For this review, use the dimensioned drawing (mm, ordinates from the lowest corner) and the shaded views. A direction names the side the tool comes from. Round coordinates to 2 decimals unless told otherwise and drop trailing zeros. Loops run counter-clockwise (first coordinate to the right, second up) from the corner with the lowest first, then second, coordinate; pieces in that order, holes last. Notation, with made-up numbers: (64.5, -18.75) -> (80.5, -18.75) arc R20 ccw to (80.5, -4.75) -> close; hole circle Ø9 at (-28.75, 34). An arc over 180 degrees is marked (long way). Write each question's results on one line, items separated by ' | '.
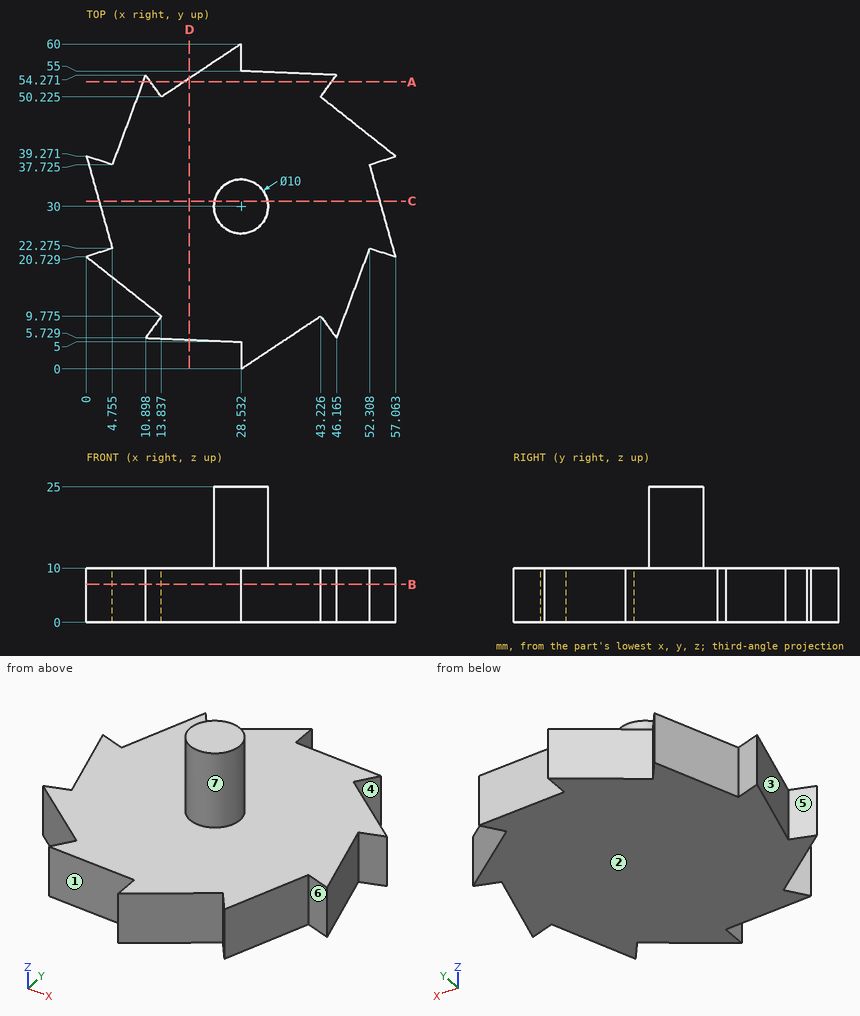
1. Consider section D-D (x = 19). State the section outline as (y, z) points (1 decimal).
Values found:
outline: (5.4, 0) -> (53.7, 0) -> (53.7, 10) -> (5.4, 10) -> close
2. Draft analysis for pull direction Y (two halves, no side actions). For the marked faces 1, 2 and 3, state which applies: released by +Y, released by -Y, zero draft, split by the parting line, or undercut.
Values found:
face 1: released by -Y | face 2: zero draft | face 3: undercut
3. For pin 1 (4 mm diameter, centred on x = 32, z = 4.5, fed in from -Y); pin 2 (4 mm diameter, centred on y = 36, z = 10, fed in from +X); pin 3 (1.5 mm diameter, centred on y = 1.5, z = 5, fed in from -X), all flat-tipped, find the tip position at first contact; note any pin that passes through.
Values found:
pin 1: stops at y = 0.98 | pin 2: stops at x = 53.35 | pin 3: stops at x = 28.53
4. Tool access review of the marked faces 4, 5, 6 and 7: name each direction out of +Z, -Z, +X, -X, +Y, -Y from which nothing blocks a thin tool from reaching the whole face with its end or side.
Values found:
face 4: +Z, -Z, +X | face 5: +Z, -Z, -X | face 6: +Z, -Z, -Y | face 7: +Z
5. Consider section A-A (y = 53). State the section outline as (x, z) points.
Values found:
outline: (10.43, 0) -> (11.82, 0) -> (11.82, 10) -> (10.43, 10) -> close; (18.01, 0) -> (45.24, 0) -> (45.24, 10) -> (18.01, 10) -> close
6. Consider section C-C (y = 31). State the section outline as (x, z) points.
Values found:
outline: (2.31, 0) -> (54.19, 0) -> (54.19, 10) -> (33.43, 10) -> (33.43, 25) -> (23.63, 25) -> (23.63, 10) -> (2.31, 10) -> close
7. Consider section B-B (z = 7). State the section outline as (x, y) points (1 decimal), plus the area to 3 significant figures.
Values found:
outline: (0, 20.7) -> (13.8, 9.8) -> (10.9, 5.7) -> (28.5, 5) -> (28.5, 0) -> (43.2, 9.8) -> (46.2, 5.7) -> (52.3, 22.3) -> (57.1, 20.7) -> (52.3, 37.7) -> (57.1, 39.3) -> (43.2, 50.2) -> (46.2, 54.3) -> (28.5, 55) -> (28.5, 60) -> (13.8, 50.2) -> (10.9, 54.3) -> (4.8, 37.7) -> (0, 39.3) -> (4.8, 22.3) -> close | area: 2,200 mm2
8. To check wall thickness, follow probe 1 along Z at (x, y) = (9.5, 22); probe 2 along X at (y, z) = (17, 4); probe 3 along X at (y, z) = (24, 7.25). State the ranges of each line that lie inside material, in increasing order.
Values found:
probe 1: z = 0 to 10 | probe 2: x = 4.71 to 50.35 | probe 3: x = 4.27 to 56.15
